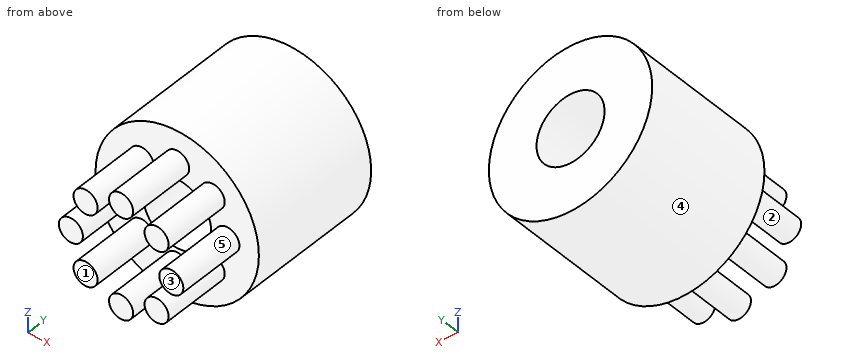
```python
from build123d import *

# Parameters (mm, degrees)
F0_R     = 30
F1_DEPTH = 50
F2_R     = 12.5
F3_DEPTH = 50.001
F4_R     = 4.418686
F5_DEPTH = 25


with BuildPart() as f1:
    # F0 (on Front) → F1 (new body)
    with BuildSketch(Plane.XZ):
        Circle(F0_R)
    extrude(amount=F1_DEPTH)

    # F2 (on face) → F3 (cut, through all)
    with BuildSketch(Plane.XZ.offset(50)):
        Circle(F2_R)
    extrude(amount=-F3_DEPTH, mode=Mode.SUBTRACT)

    # F4 (on face) → F5 (join)
    with BuildSketch(Plane.XZ.offset(50)):
        with Locations((18.444646, 0)):
            Circle(F4_R)
        with Locations((13.042334, 13.042334)):
            Circle(F4_R)
        with Locations((0, 18.444646)):
            Circle(F4_R)
        with Locations((-13.042334, 13.042334)):
            Circle(F4_R)
        with Locations((-18.444646, 0)):
            Circle(F4_R)
        with Locations((-13.042334, -13.042334)):
            Circle(F4_R)
        with Locations((0, -18.444646)):
            Circle(F4_R)
        with Locations((13.042334, -13.042334)):
            Circle(F4_R)
    extrude(amount=F5_DEPTH)


solid = f1.part
```
Work out the finished part from the listing and answer in its coordinate system (mm). Face numbers are marked on the shaded views. A direction names the side the tool comes from. Coordinates: 2 decimals unless noted, no trailing zeros. Order: outer loops, then holes, each group sorted by start corner. A loop starts at its lowest first (then second) coordinate and runs counter-clockwise, first axis right, second up. Notation, with made-up numbers: M 27,9 L 41,9 A21 cw 41,14 Z; hole C 52.25,-30 d7. An arc over 180 degrees is marked long. Use CSV: the item, a comma, the result in double quotes.
1) Section A-A on z = 0 is taken. Write down the section's boundary in (x, y), plus the area to 3 significant figures.
Worked out:
outline,"M -30,-50 L -22.86,-50 L -22.86,-75 L -14.03,-75 L -14.03,-50 L -12.5,-50 L -12.5,0 L -30,0 Z; M 12.5,-50 L 14.03,-50 L 14.03,-75 L 22.86,-75 L 22.86,-50 L 30,-50 L 30,0 L 12.5,0 Z"
area,"2,190 mm^2"
2) Section C-C on y = -47 is taken. Write down the section's boundary in (x, z), plus the area to 3 significant figures.
Worked out:
outline,"C 0,0 d60; hole C 0,0 d25"
area,"2,340 mm^2"
3) Section D-D on z = 7 is taken. Write down the section's boundary in (x, y).
Worked out:
outline,"M -29.17,-50 L -10.36,-50 L -10.36,0 L -29.17,0 Z; M 10.36,-50 L 29.17,-50 L 29.17,0 L 10.36,0 Z"
4) Consider line 1 (Z direction, x = 0, y = -15); line 2 (Y direction, x = -10.5, z = 8.5); line 3 (Z direction, x = -16, y = -56.5). Determine where each line is inside the solid, lowest interval first. Write a range as [from, to].
Worked out:
line 1,"z = [-30, -12.5], [12.5, 30]"
line 2,"y = [-50, 0]"
line 3,"z = [-16.33, -9.76], [-3.68, 3.68], [9.76, 16.33]"
5) Flat-ended cylindrical pins translate along their axes: pin 1 Ø4 at (y, z) = (-33.5, -23) entering from -X; pin 2 Ø3 at (y, z) = (-37.5, 14) entering from -X; pin 3 Ø6 at (y, z) = (-36.5, 23) entering from -X. Find the tip coordinate at first contact, or state that the pin passes through.
Worked out:
pin 1,"stops at x = -21.42"
pin 2,"stops at x = -27.27"
pin 3,"stops at x = -22.36"
6) Section B-B on x = 0 is taken. Write down the section's boundary in (y, z), plus the area to 3 significant figures.
Worked out:
outline,"M -75,-22.86 L -50,-22.86 L -50,-30 L 0,-30 L 0,-12.5 L -50,-12.5 L -50,-14.03 L -75,-14.03 Z; M -75,14.03 L -50,14.03 L -50,12.5 L 0,12.5 L 0,30 L -50,30 L -50,22.86 L -75,22.86 Z"
area,"2,190 mm^2"
7) For the marked faces 1 and 2, determine the directions among +Z, -Z, +X, -X, +Y, -Y from which every point of the face is accessible in a straight line to the end or side of a thin tool.
Worked out:
face 1,"+Z, -Z, +X, -X, -Y"
face 2,"-Y"
8) Determine the mould class of the marked faces 3, 4 and 5 for opening direction Z: released by +Z, released by -Z, zero draft, split by the parting line, or undercut.
Worked out:
face 3,"zero draft"
face 4,"split by the parting line"
face 5,"undercut"
